Work out the finished part from the listing and answer in its coordinate system (mm). A direction names the side the tool comes from. Round coordinates to 2 decimals unless told otherwise and drop trailing zeros. Write each loop counter-clockwise with the first axis right and the second up, starting at its lowest first coordinate (ties: lowest second). Pieces come first, ordered by that corner, then holes.
1. Find section B-B (x = -15.5). Write down the section's boundary in (y, z), and give its area (3 significant figures).
2. Find section C-C (y = 70). Write down the section's boundary in (x, z), and give its area (3 significant figures).
3. Find section A-A (z = -7.5). Write down the section's boundary in (x, y), and give its area (3 significant figures).
4. Flat-ended cylindrical pins translate along their axes: pin 1 Ø12 at (y, z) = (159.5, -26.5) entering from -X; pin 2 Ø5 at (x, y) = (-30, 23) entering from +Z; pin 3 Ø4 at (x, y) = (15, 55) entering from +Z; pin 4 Ø4 at (y, z) = (44, -39) entering from -X. Find the tip coordinate at first contact, or state that the pin passes through.
5. A tool of negligible diameter and unlimited length cuts with its end or side. For faces 1 (the face through (0.945, 127.962, -6.261)), 2 (the face through (-11, 203.2, -48)), from which of +Z, -Z, +X, -X, +Y, -Y can it reach the whole face along a straight path? Write none if from no direction.
6. Determine the mould class of faces 3 (the face through (-11, 0, -48)), 4 (the face through (42.75, 100.18, -46.37)), 5 (the face through (-10, 60, -12.7)) for opening direction Y: pulls with the +Y half, pulls with the -Y half, needs draft (parallel to the pull), parting line crosses it, or undercut.
7. Find section D-D (x = 6). Write down the section's boundary in (y, z).
8. Straight lines are drawn through the part: probe 1 along Z at (x, y) = (-14, 168.5); probe 2 along X at (y, z) = (121, -75); probe 3 along X at (y, z) = (22, -64). For each, find the intervals that lie inside material, in ascending order.
```python
from build123d import *

# Parameters (mm, degrees)
BOSS_EXTRUDE1_DEPTH = 203.2
SKETCH2_R           = 23.365349899
SKETCH2_R_2         = 41.378531947
CUT_EXTRUDE1_DEPTH  = 12.7


with BuildPart() as part:
    # Sketch1 → Boss-Extrude1 (new body)
    with BuildSketch(Plane(origin=(0, 0, 0), x_dir=(1, 0, 0), z_dir=(0, 1, 0))):
        Polygon((-76.511565421, 0), (56.838434579, 0), (28.263434579, 94.053387857), (-47.936565421, 94.053387857), align=None)
    extrude(amount=BOSS_EXTRUDE1_DEPTH)

    # Sketch2 → Cut-Extrude1 (cut)
    with BuildSketch(Plane.XY):
        with Locations((-9.836565421, 148.691225426)):
            Circle(SKETCH2_R)
        with Locations((-9.836565421, 59.601825969)):
            Circle(SKETCH2_R_2)
    extrude(amount=-CUT_EXTRUDE1_DEPTH, mode=Mode.SUBTRACT)


solid = part.part
```
Worked answers:
1. outline: (0, -94.05) - (203.2, -94.05) - (203.2, 0) - (171.36, 0) - (171.36, -12.7) - (126.02, -12.7) - (126.02, 0) - (100.59, 0) - (100.59, -12.7) - (18.61, -12.7) - (18.61, 0) - (0, 0) - close
1. area: 17,500 mm2
2. outline: (-76.51, 0) - (-47.94, -94.05) - (28.26, -94.05) - (56.84, 0) - (30.21, 0) - (30.21, -12.7) - (-49.89, -12.7) - (-49.89, 0) - close
2. area: 8,840 mm2
3. outline: (-74.23, 0) - (54.56, 0) - (54.56, 203.2) - (-74.23, 203.2) - close; hole circle Ø82.76 at (-9.84, 59.6); hole circle Ø46.73 at (-9.84, 148.69)
3. area: 19,100 mm2
4. pin 1: stops at x = -70.28
4. pin 2: stops at z = 0
4. pin 3: stops at z = -12.7
4. pin 4: stops at x = -65.27
5. face 1: +Z
5. face 2: +Z, -Z, +X, -X, +Y
6. face 3: pulls with the -Y half
6. face 4: needs draft
6. face 5: undercut
7. outline: (0, -94.05) - (203.2, -94.05) - (203.2, 0) - (165.87, 0) - (165.87, -12.7) - (131.51, -12.7) - (131.51, 0) - (97.83, 0) - (97.83, -12.7) - (21.37, -12.7) - (21.37, 0) - (0, 0) - close
8. probe 1: z = -94.05 to -12.7
8. probe 2: x = -53.73 to 34.05
8. probe 3: x = -57.07 to 37.39
